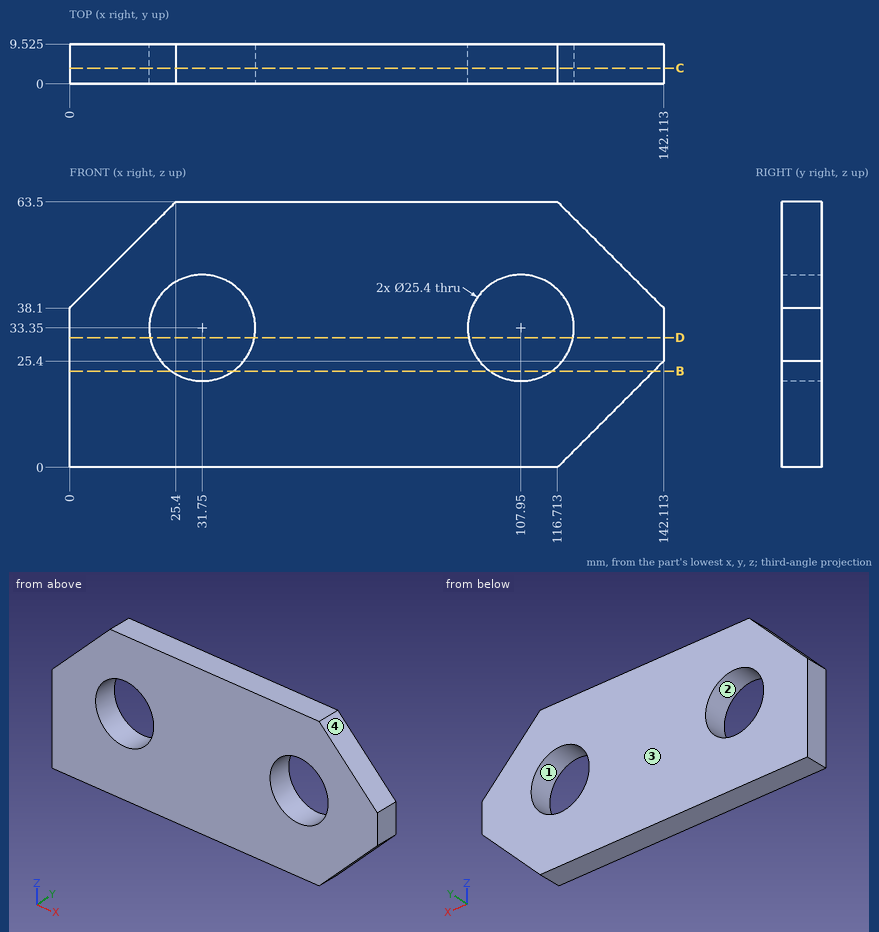
The drawing under review shows one solid part. Ordinate dimensions are in mm from its lowest x, y, z. Round coordinates to 2 decimals unless told otherwise and drop trailing zeros. Order: outer loops, then holes, each group sorted by start corner. A loop starts at its lowest first (then second) coordinate and runs counter-clockwise, first axis right, second up. Notation, with made-up numbers: M 10.25,22.25 L 31.25,22.25 A27 cw 31.25,39.25 Z; hole C 66,-25.5 d9. An arc over 180 degrees is marked long. Answer as CSV lines item,"result". Start each with the question number.
1) The part is to be moulded in two halves that separate along Z. For the marked faces 1, 2, 3 and 4, say which applies: +Z half, -Z half, draft (parallel to the pull), parting line (faces both ways), or undercut.
2) Add section B-B (z = 23). Give the boundary of the cut face in (x, y) (1 decimal), then the cut area to 3 significant figures.
3) Add section C-C (y = 3.75). Give the boundary of the cut face in (x, z).
4) Wall thickness on line 1 along Z through (x, y) = (107.95, 7.5); line 2 along X through (y, z) = (1, 30.5); line 3 along X through (y, z) = (4.5, 38.5): over which ranges is each line inside the solid? List them lowest first. Write a range as [from, to].
5) For pin 1 Ø2 at (y, z) = (1.5, 56.5) entering from -X; pin 2 Ø15 at (x, z) = (107.95, 33.35) entering from +Y; pin 3 Ø5 at (y, z) = (4.5, 13.5) entering from +X; pin 4 Ø3 at (x, y) = (19.5, 7.5) entering from +Z, all flat-tipped, find the tip position at first contact; note any pin that passes through.
6) Add section D-D (z = 31). Give the boundary of the cut face in (x, y) (1 decimal).
Resolved:
1,face 1,"undercut"
1,face 2,"undercut"
1,face 3,"draft"
1,face 4,"+Z half"
2,outline,"M 0,0 L 24.4,0 L 24.4,9.5 L 0,9.5 Z; M 39.1,0 L 100.6,0 L 100.6,9.5 L 39.1,9.5 Z; M 115.3,0 L 139.7,0 L 139.7,9.5 L 115.3,9.5 Z"
2,area,"1,050 mm^2"
3,outline,"M 0,0 L 116.71,0 L 142.11,25.4 L 142.11,38.1 L 116.71,63.5 L 25.4,63.5 L 0,38.1 Z; hole C 31.75,33.35 d25.4; hole C 107.95,33.35 d25.4"
4,line 1,"[0, 20.65], [46.05, 63.5]"
4,line 2,"[0, 19.37], [44.13, 95.57], [120.33, 142.11]"
4,line 3,"[0.4, 20.14], [43.36, 96.34], [119.56, 141.71]"
5,pin 1,"x = 17.4"
5,pin 2,"through"
5,pin 3,"x = 132.71"
5,pin 4,"z = 59.1"
6,outline,"M 0,0 L 19.3,0 L 19.3,9.5 L 0,9.5 Z; M 44.2,0 L 95.5,0 L 95.5,9.5 L 44.2,9.5 Z; M 120.4,0 L 142.1,0 L 142.1,9.5 L 120.4,9.5 Z"
